Design review of the part shown in the three views and the two pictorial views. Dimensions are in mm from the part's minimum x, y and z. A direction names the side the tool comes from. Coordinates: 2 decimals unless noted, no trailing zeros. Loops run counter-clockwise (first coordinate to the right, second up) from the corner with the lowest first, then second, coordinate; pieces in that order, holes last. Notation, with made-up numbers: (13.5, 57) -> (35.5, 57) arc R28 ccw to (35.5, 94) -> close; hole circle Ø4 at (-32.5, 54.25). An arc over 180 degrees is marked (long way). One line per item, written item: value. Start each with the question number.
1. Add section B-B on z = 2. Write out the cut boundary in (x, y).
2. Add section D-D on y = 7.25. Write out the cut boundary in (x, z), plus the area to 3 significant figures.
3. Insertion check: pin 1 (0.8 mm diameter, centred on x = 6, z = 2, fed in from -Y); pin 2 (1.5 mm diameter, centred on y = 8, z = 3, fed in from -X). Each pin has a flat end and moves straight along its axis. Give the tip position at first contact, or say it passes through.
4. Draft analysis for pull direction Z (two halves, no side actions). For the marked faces 1, 2, 3 and 4, state which applies: pulls with the +Z half, pulls with the -Z half, needs draft (parallel to the pull), parting line crosses it, or undercut.
5. Add section A-A on y = 3.5. Write out the cut boundary in (x, z).
6. For probe 1 along Z at (x, y) = (26, 3.7); probe 2 along X at (y, z) = (3.5, 1); probe 3 along X at (y, z) = (4, 1.5), list the stretches that pass through material, from the lowest coordinate up.
7. Add section C-C on x = 2. Write out the cut boundary in (y, z).
8. Machinability: for the marked faces 5 and 6, which of the approach directions +Z, -Z, +X, -X, +Y, -Y give a long, thin tool a straight path to every point of the face, cutting with its end or side? Answer none if there is none.
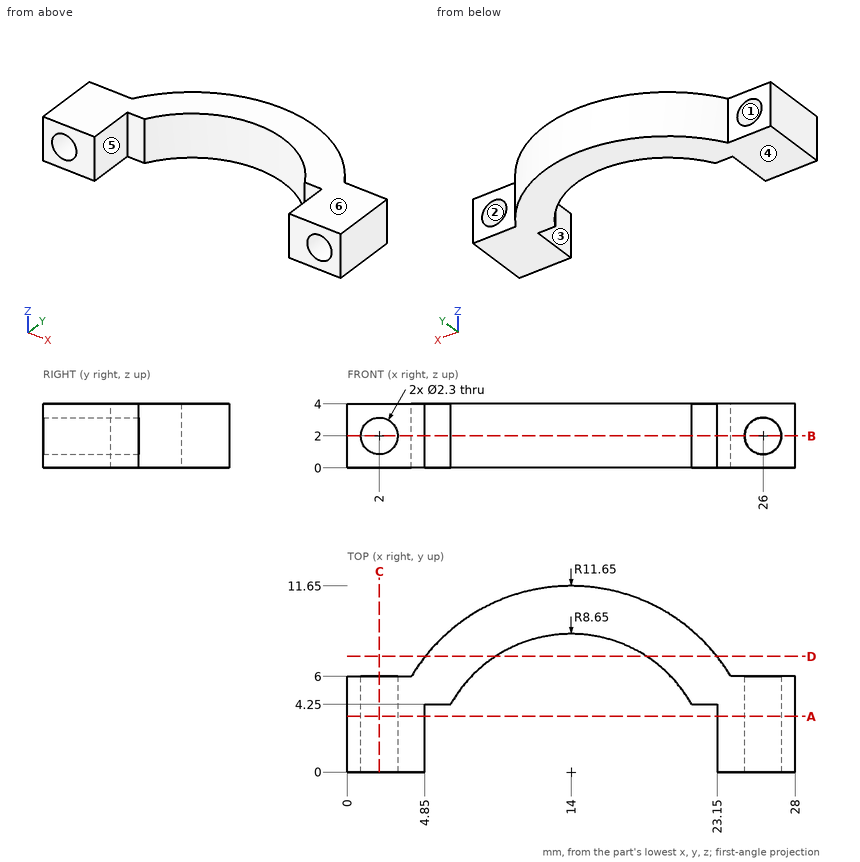
Worked answers:
1. outline: (0, 0) -> (0.85, 0) -> (0.85, 6) -> (0, 6) -> close; (3.15, 0) -> (4.85, 0) -> (4.85, 4.25) -> (6.47, 4.25) arc R8.65 cw to (21.53, 4.25) -> (23.15, 4.25) -> (23.15, 0) -> (24.85, 0) -> (24.85, 6) -> (23.99, 6) arc R11.65 ccw to (4.01, 6) -> (3.15, 6) -> close; (27.15, 0) -> (28, 0) -> (28, 6) -> (27.15, 6) -> close
2. outline: (4.88, 0) -> (9.28, 0) -> (9.28, 4) -> (4.88, 4) -> close; (18.72, 0) -> (23.12, 0) -> (23.12, 4) -> (18.72, 4) -> close
2. area: 35.2 mm²
3. pin 1: stops at y = 4.25
3. pin 2: stops at x = 4.88
4. face 1: undercut
4. face 2: undercut
4. face 3: needs draft
4. face 4: pulls with the -Z half
5. outline: (0, 0) -> (4.85, 0) -> (4.85, 4) -> (0, 4) -> close; (23.15, 0) -> (28, 0) -> (28, 4) -> (23.15, 4) -> close; hole circle Ø2.3 at (2, 2); hole circle Ø2.3 at (26, 2)
6. probe 1: z = 0 to 0.85, 3.15 to 4
6. probe 2: x = 0 to 1.43, 2.57 to 4.85, 23.15 to 25.43, 26.57 to 28
6. probe 3: x = 0 to 0.96, 3.04 to 4.85, 23.15 to 24.96, 27.04 to 28
7. outline: (0, 0) -> (6, 0) -> (6, 0.85) -> (0, 0.85) -> close; (0, 3.15) -> (6, 3.15) -> (6, 4) -> (0, 4) -> close
8. face 5: +Z, -Z, -Y
8. face 6: +Z, +X, -X, +Y, -Y
